The model under review builds one solid part; all positions refer to its coordinate system, in mm. A direction names the side the tool comes from. Coordinates: 2 decimals unless noted, no trailing zeros. Write each loop counter-clockwise with the first axis right and the second up, starting at its lowest first coordinate (ties: lowest second). Pieces come first, ordered by that corner, then holes. Notation, with made-up numbers: (-2, 62) - (52, 62) arc R23 ccw to (52, 77) - close; hole circle Ø9 at (4.5, 49). An arc over 180 degrees is marked (long way). Use one line per item in the form item = value. Start each with the question number.
```python
from build123d import *

# Parameters (mm, degrees)
BOSS_EXTRU_1_DEPTH         = 10
ESQUISSE2_W                = 10
ESQUISSE2_H                = 10
ENL_V_MAT_EXTRU_1_DEPTH    = 10
R_P_TITION_LIN_AIRE1_COUNT = 3
R_P_TITION_LIN_AIRE1_PITCH = 20
ESQUISSE3_W                = 10
ESQUISSE3_H                = 10
ENL_V_MAT_EXTRU_2_DEPTH    = 10
R_P_TITION_LIN_AIRE2_COUNT = 4
R_P_TITION_LIN_AIRE2_PITCH = 20
ENL_V_MAT_EXTRU_3_DEPTH    = 10
ESQUISSE5_R                = 5
ENL_V_MAT_EXTRU_4_DEPTH    = 10


with BuildPart() as part:
    # Esquisse1 → Boss.-Extru.1 (new body)
    with BuildSketch(Plane.XY):
        Polygon((0, 0), (-30, 0), (-30, 227), (-143, 227), (-143, 300), (0, 300), align=None)
    extrude(amount=BOSS_EXTRU_1_DEPTH)

    # Esquisse2 → Enlèv. mat.-Extru.1 (cut)
    with BuildSketch(Plane.XY.offset(10)):
        with Locations((-138, 295)):
            Rectangle(ESQUISSE2_W, ESQUISSE2_H)
    enl_v_mat_extru_1 = extrude(amount=-ENL_V_MAT_EXTRU_1_DEPTH, mode=Mode.SUBTRACT)

    # Répétition linéaire1: Enlèv. mat.-Extru.1 ×3
    with Locations(*[(0, -i * R_P_TITION_LIN_AIRE1_PITCH, 0) for i in range(1, R_P_TITION_LIN_AIRE1_COUNT)]):
        add(enl_v_mat_extru_1, mode=Mode.SUBTRACT)

    # Esquisse3 → Enlèv. mat.-Extru.2 (cut)
    with BuildSketch(Plane.XY.offset(10)):
        with Locations((-25, 162)):
            Rectangle(ESQUISSE3_W, ESQUISSE3_H)
    enl_v_mat_extru_2 = extrude(amount=-ENL_V_MAT_EXTRU_2_DEPTH, mode=Mode.SUBTRACT)

    # Répétition linéaire2: Enlèv. mat.-Extru.2 ×4
    with Locations(*[(0, -i * R_P_TITION_LIN_AIRE2_PITCH, 0) for i in range(1, R_P_TITION_LIN_AIRE2_COUNT)]):
        add(enl_v_mat_extru_2, mode=Mode.SUBTRACT)

    # Esquisse4 → Enlèv. mat.-Extru.3 (cut)
    with BuildSketch(Plane.XY.offset(10)):
        with BuildLine():
            Line((-4, 221), (-4, 171))
            ThreePointArc((-4, 171), (-10, 165), (-16, 171))
            Line((-16, 171), (-16, 221))
            ThreePointArc((-16, 221), (-10, 227), (-4, 221))
        make_face()
    extrude(amount=-ENL_V_MAT_EXTRU_3_DEPTH, mode=Mode.SUBTRACT)

    # Esquisse5 → Enlèv. mat.-Extru.4 (cut)
    with BuildSketch(Plane.XY.offset(10)):
        with Locations((-58.415926493, 235.370461514)):
            Circle(ESQUISSE5_R)
    extrude(amount=-ENL_V_MAT_EXTRU_4_DEPTH, mode=Mode.SUBTRACT)


solid = part.part
```
1. The part is to be moulded in two halves that separate along X. For faces 1 (the flat face through (-4, 196, 5)), 2 (the flat face through (-143, 238, 5)), 3 (the flat face through (-25, 117, 5)), say which applies: released by +X, released by -X, zero draft, split by the parting line, or undercut.
2. For faces 4 (the flat face through (-30, 197, 5)), 5 (the cylindrical face through (-10, 227, 5)), 6 (the flat face through (-25, 157, 5)), 7 (the flat face through (-138, 290, 5)), 8 (the flat face through (-67, 300, 5)), list the 3-axis set-ups (+Z, -Z, +X, -X, +Y, -Y) from which the entire face can be reached by the end or side of a thin tool; tool diameter is ignored.
3. Take a section at A-A (x = -10). State the section outline as (y, z) points.
4. Take a section at C-C (x = -67.5). State the section outline as (y, z) points, plus the area to 3 significant figures.
5. For P1, Ø1.5, axis at y = 94.5, z = 7.5, coming from the +X side; P2, Ø5, axis at y = 113, z = 7, coming from the -X side; P3, Ø5, axis at x = -139, z = 3.5, coming from the -Y side; P4, Ø2, axis at y = 104, z = 6, coming from the -X side, all flat-tipped, find the tip position at first contact; note any pin that passes through.
6. For L1, parallel to X at y = 201, z = 6.25; L2, parallel to Y at x = -29, z = 4; L3, parallel to Y at x = -58.5, z = 7, list the stretches that pass through material, from the lowest coordinate up.
7. Take a section at D-D (z = 3.25). Count the separate pieces of the cut face and the enclosed holes in it, plus the area to 3 significant figures.
8. Take a section at B-B (y = 120.5). State the section outline as (x, z) points, plus the area to 3 significant figures.
Returned:
q1.face_1 = undercut
q1.face_2 = released by -X
q1.face_3 = zero draft
q2.face_4 = +Z, -Z, -X, -Y
q2.face_5 = +Z, -Z
q2.face_6 = +Z, -Z, -X
q2.face_7 = +Z, -Z, -X, +Y
q2.face_8 = +Z, -Z, +X, -X, +Y
q3.outline = (0, 0) - (165, 0) - (165, 10) - (0, 10) - close; (227, 0) - (300, 0) - (300, 10) - (227, 10) - close
q4.outline = (227, 0) - (300, 0) - (300, 10) - (227, 10) - close
q4.area = 730 mm²
q5.P1 = 0
q5.P2 = -30
q5.P3 = 227
q5.P4 = -20
q6.L1 = -30 to -16, -4 to 0
q6.L2 = 0 to 97, 107 to 117, 127 to 137, 147 to 157, 167 to 300
q6.L3 = 227 to 230.37, 240.37 to 300
q7.separate_pieces = 1
q7.enclosed_holes = 2
q7.area = 15,800 mm²
q8.outline = (-20, 0) - (0, 0) - (0, 10) - (-20, 10) - close
q8.area = 200 mm²
